```python
from build123d import *

# Parameters (mm, degrees)
F1_DEPTH = 9
F0_R     = 2.5
F0_R_2   = 51.75
F2_DEPTH = 4.5
F3_R     = 11
F0_R_3   = 1.25
F4_DEPTH = 6


with BuildPart() as f1:
    # F0 (on Right) → F1 (new body)
    with BuildSketch(Plane.YZ):
        Polygon((67.5, -115), (67.5, 115), (0, 115), (-67.5, 115), (-67.5, -115), align=None)
        with BuildLine():
            ThreePointArc((-47.0226009489, -3.9773990511), (-24.0347326375, 3.4781900517), (0, 6))
            ThreePointArc((0, 6), (24.0347326375, 3.4781900517), (47.0226009489, -3.9773990511))
            ThreePointArc((47.0226009489, -3.9773990511), (57, -51), (47.0226009489, -98.0226009489))
            ThreePointArc((47.0226009489, -98.0226009489), (0, -108), (-47.0226009489, -98.0226009489))
            ThreePointArc((-47.0226009489, -98.0226009489), (-57, -51), (-47.0226009489, -3.9773990511))
        make_face(mode=Mode.SUBTRACT)
        with BuildLine():
            ThreePointArc((0, 10.1854634317), (-50.3290897047, 60.4354011911), (0, 110.6853389504))
            ThreePointArc((0, 110.6853389504), (35.4809774891, 95.9395435011), (50.1709102953, 60.4354011911))
            ThreePointArc((50.1709102953, 60.4354011911), (35.4809774891, 24.9312588811), (0, 10.1854634317))
        make_face(mode=Mode.SUBTRACT)
    extrude(amount=-F1_DEPTH)

    # F0 (on Right) → F2 (join)
    with BuildSketch(Plane.YZ):
        with BuildLine():
            ThreePointArc((47.0226009489, -3.9773990511), (24.0347326375, 3.4781900517), (0, 6))
            ThreePointArc((0, 6), (-24.0347326375, 3.4781900517), (-47.0226009489, -3.9773990511))
            ThreePointArc((-47.0226009489, -3.9773990511), (-57, -51), (-47.0226009489, -98.0226009489))
            ThreePointArc((-47.0226009489, -98.0226009489), (0, -108), (47.0226009489, -98.0226009489))
            ThreePointArc((47.0226009489, -98.0226009489), (57, -51), (47.0226009489, -3.9773990511))
        make_face()
        with Locations((-40.3050865276, -91.3050865276)):
            Circle(F0_R, mode=Mode.SUBTRACT)
        with Locations((-40.3050865276, -10.6949134724)):
            Circle(F0_R, mode=Mode.SUBTRACT)
        with Locations((40.3050865276, -91.3050865276)):
            Circle(F0_R, mode=Mode.SUBTRACT)
        with Locations((0, -51)):
            Circle(F0_R_2, mode=Mode.SUBTRACT)
        with Locations((40.3050865276, -10.6949134724)):
            Circle(F0_R, mode=Mode.SUBTRACT)
    extrude(amount=-F2_DEPTH)

    # F3
    f3_edges = [f1.edges().sort_by_distance(p)[0] for p in [
        (-6.75, 47.022601, -3.977399),
        (-6.75, -47.022601, -3.977399),
        (-6.75, -47.022601, -98.022601),
        (-6.75, 47.022601, -98.022601),
    ]]
    fillet(f3_edges, radius=F3_R)

    # F0 (on Right) → F4 (join)
    with BuildSketch(Plane.YZ):
        with BuildLine():
            ThreePointArc((50.1709102953, 60.4354011911), (35.4809774891, 95.9395435011), (0, 110.6853389504))
            Line((0, 110.6853389504), (0, 99.4354011911))
            Line((0, 99.4354011911), (18.9209102953, 99.4354011911))
            ThreePointArc((18.9209102953, 99.4354011911), (21.0422306388, 98.5567215346), (21.9209102953, 96.4354011911))
            Line((21.9209102953, 96.4354011911), (21.9209102953, 24.4354011911))
            ThreePointArc((21.9209102953, 24.4354011911), (21.0422306388, 22.3140808475), (18.9209102953, 21.4354011911))
            Line((18.9209102953, 21.4354011911), (0, 21.4354011911))
            Line((0, 21.4354011911), (0, 10.1854634317))
            ThreePointArc((0, 10.1854634317), (35.4809774891, 24.9312588811), (50.1709102953, 60.4354011911))
        make_face()
        with Locations((28.8463527312, 25.9634012507)):
            Circle(F0_R_3, mode=Mode.SUBTRACT)
        with Locations((28.8463527312, 94.9074011314)):
            Circle(F0_R_3, mode=Mode.SUBTRACT)
        with Locations((45.0773127377, 60.3711940348)):
            Circle(F0_R_3, mode=Mode.SUBTRACT)
        with BuildLine():
            Line((0, 99.4354011911), (0, 110.6853389504))
            ThreePointArc((0, 110.6853389504), (-50.3290897047, 60.4354011911), (0, 10.1854634317))
            Line((0, 10.1854634317), (0, 21.4354011911))
            Line((0, 21.4354011911), (-19.0790897047, 21.4354011911))
            ThreePointArc((-19.0790897047, 21.4354011911), (-21.2004100483, 22.3140808475), (-22.0790897047, 24.4354011911))
            Line((-22.0790897047, 24.4354011911), (-22.0790897047, 96.4354011911))
            ThreePointArc((-22.0790897047, 96.4354011911), (-21.2004100483, 98.5567215346), (-19.0790897047, 99.4354011911))
            Line((-19.0790897047, 99.4354011911), (0, 99.4354011911))
        make_face()
        with Locations((-28.8463527312, 25.9634012507)):
            Circle(F0_R_3, mode=Mode.SUBTRACT)
        with Locations((-45.6305965781, 60.3711940348)):
            Circle(F0_R_3, mode=Mode.SUBTRACT)
        with Locations((-28.8463527312, 94.9074011314)):
            Circle(F0_R_3, mode=Mode.SUBTRACT)
    extrude(amount=-F4_DEPTH)


solid = f1.part
```
Read the model definition and answer for the solid it produces. Units are mm, in the model's axes. A direction names the side the tool comes from. Give positions to 0.01 mm unless a question says otherwise; leave off trailing zeros. Write each loop counter-clockwise with the first axis right and the second up, starting at its lowest first coordinate (ties: lowest second). Pieces come first, ordered by that corner, then holes. Notation, with made-up numbers: M 17.25,70 L 70.25,70 A17 cw 70.25,97 Z; hole C 60.25,61 d7. An arc over 180 degrees is marked long. Put each result on its own line as item: value. Start each with the question number.
1. The part is cut by section A-A, the plane z = -51. Give the vertices of the cut face in (x, y).
2. For a pull along Z with two mould halves and no side action, classify faces 1 (the flat face through (-4, -67.5, 2)), 2 (the flat face through (-3, 0, 99.435)), 3 (the flat face through (-4, 1, 115)) as released by +Z, released by -Z, zero draft, split by the parting line, or undercut.
3. Each of these flat-tipped pins is pushed along its axis until it touches: pin 1 Ø6.5 at (y, z) = (-40.31, -10.69) entering from -X; pin 2 Ø4 at (y, z) = (40.31, -10.69) entering from -X (3 decimals); pin 3 Ø3 at (y, z) = (28.85, 25.96) entering from -X. Where does it stop, or does it pass through?
4. The part is cut by section C-C, the plane z = -27.5. Give the vertices of the cut face in (x, y).
5. Consider line 1 along Y through (x, z) = (-2, 81); line 2 along Z through (x, y) = (-7.5, 1.5); line 3 along Y through (x, z) = (-1.25, 59.5). Determine where each line is inside the solid, lowest interval first.
6. The part is cut by section D-D, the plane y = -13. Give the vertices of the cut face in (x, z) (3 decimals), and give its area (3 significant figures).
7. Which of the six approach directions +Z, -Z, +X, -X, +Y, -Y give full straight-line access (tool end or side, diameter ignored) to faces 4 (the flat face through (-3, -22.079, 60)), 5 (the flat face through (0, -1, 2)), 6 (the cylindrical face through (-6.7, -57, -51.6))?
8. The part is cut by section B-B, the plane y = 13.5. Give the vertices of the cut face in (x, z), and give its area (3 significant figures).
Final values:
1. outline: M -9,-67.5 L 0,-67.5 L 0,-51.75 L -4.5,-51.75 L -4.5,-57 L -9,-57 Z; M -9,57 L -4.5,57 L -4.5,51.75 L 0,51.75 L 0,67.5 L -9,67.5 Z
2. face 1: zero draft
2. face 2: undercut
2. face 3: released by +Z
3. pin 1: stops at x = -4.5
3. pin 2: passes through
3. pin 3: stops at x = -6
4. outline: M -9,-67.5 L 0,-67.5 L 0,-46.11 L -4.5,-46.11 L -4.5,-54.59 L -9,-54.59 Z; M -9,54.59 L -4.5,54.59 L -4.5,46.11 L 0,46.11 L 0,67.5 L -9,67.5 Z
5. line 1: y = -67.5 to -22.08, 21.92 to 67.5
5. line 2: z = -115 to -107.99, 5.99 to 10.21, 110.66 to 115
5. line 3: y = -67.5 to -46.53, -44.73 to -22.08, 21.92 to 44.18, 45.97 to 67.5
6. outline: M -9,-115 L 0,-115 L 0,-101.091 L -4.5,-101.091 L -4.5,-107.268 L -9,-107.268 Z; M -9,5.268 L -4.5,5.268 L -4.5,-0.909 L 0,-0.909 L 0,21.435 L -6,21.435 L -6,11.875 L -9,11.875 Z; M -9,108.996 L -6,108.996 L -6,99.435 L 0,99.435 L 0,115 L -9,115 Z
6. area: 353 mm²
7. face 4: +X, -X
7. face 5: +Z, -Z, +X, +Y, -Y
7. face 6: -X
8. outline: M -9,-115 L 0,-115 L 0,-100.96 L -4.5,-100.96 L -4.5,-107.21 L -9,-107.21 Z; M -9,5.21 L -4.5,5.21 L -4.5,-1.04 L 0,-1.04 L 0,21.44 L -6,21.44 L -6,12.05 L -9,12.05 Z; M -9,108.82 L -6,108.82 L -6,99.44 L 0,99.44 L 0,115 L -9,115 Z
8. area: 356 mm²
